Check sheet for the modelled part. Datum: model origin and axes. Units: mm. Round coordinates to 2 decimals unless told otherwise and drop trailing zeros. Write each loop counter-clockwise with the first axis right and the second up, starting at its lowest first coordinate (ties: lowest second). Pieces come first, ordered by that corner, then holes. Notation, with made-up numbers: (88.25, -8) - (137.25, -8) arc R11 cw to (137.25, 11) - close; hole circle Ø7 at (26, -15.5). An arc over 180 degrees is marked (long way). Answer as a JSON object with one key per item and string values. Group by question number.
Item 1: Thickness scan on line 1 (X direction, y = 13, z = 17.75); line 2 (X direction, y = 18, z = 13.75); line 3 (Z direction, x = 5.5, y = 15.5). Record the ranges inside material, lowest first.
Item 2: Sectioned sample at B-B on x = 5. Record the boundary of the cut face in (y, z), plus the area to 3 significant figures.
Item 3: Sectioned sample at A-A on z = 14.75. Record the boundary of the cut face in (x, y).
Item 4: Sectioned sample at C-C on y = 10.5. Record the boundary of the cut face in (x, z).
Item 5: Gauge pin test, flat ends, axial feed: P1, Ø1, axis at y = 11, z = 6, coming from the +X side; P2, Ø1, axis at y = 14, z = 12, coming from the -X side; P3, Ø2, axis at x = 15.5, y = 12.5, coming from the -Z side. Record the tip position at first contact, or that the pin passes through.
```python
from build123d import *

# Parameters (mm, degrees)
SKETCH1_W           = 20
SKETCH1_H           = 20
BOSS_EXTRUDE1_DEPTH = 20
CUT_EXTRUDE1_DEPTH  = 20
CUT_EXTRUDE2_DEPTH  = 20


with BuildPart() as part:
    # Sketch1 → Boss-Extrude1 (new body)
    with BuildSketch(Plane.XY):
        with Locations((10, 10)):
            Rectangle(SKETCH1_W, SKETCH1_H)
    extrude(amount=BOSS_EXTRUDE1_DEPTH)

    # Sketch2 → Cut-Extrude1 (cut)
    with BuildSketch(Plane(origin=(0, 20, 0), x_dir=(1, 0, 0), z_dir=(0, 1, 0))):
        Polygon((20, 0), (10, 0), (20, -10), align=None)
    extrude(amount=-CUT_EXTRUDE1_DEPTH, mode=Mode.SUBTRACT)

    # Sketch3 → Cut-Extrude2 (cut)
    with BuildSketch(Plane(origin=(0, 20, 0), x_dir=(1, 0, 0), z_dir=(0, 1, 0))):
        Polygon((20, -20), (0, -20), (0, -10), align=None)
    extrude(amount=-CUT_EXTRUDE2_DEPTH, mode=Mode.SUBTRACT)


solid = part.part
```
Completed:
{
 "1": {"line 1": "15.5 to 20", "line 2": "7.5 to 20", "line 3": "0 to 12.75"},
 "2": {"outline": "(0, 0) - (20, 0) - (20, 12.5) - (0, 12.5) - close", "area": "250 mm²"},
 "3": {"outline": "(9.5, 0) - (20, 0) - (20, 20) - (9.5, 20) - close"},
 "4": {"outline": "(0, 0) - (10, 0) - (20, 10) - (20, 20) - (0, 10) - close"},
 "5": {"P1": "x = 16.5", "P2": "x = 3", "P3": "z = 4.5"}
}
